```python
from build123d import *

# Parameters (mm, degrees)
F0_W     = 40
F0_H     = 20
F1_DEPTH = 6
F2_W     = 16
F2_H     = 12
F2_R     = 4.65
F3_DEPTH = 3
F4_DEPTH = 1.5
F5_SIZE  = 1


with BuildPart() as f1:
    # F0 (on Top) → F1 (new body)
    with BuildSketch(Plane.XY):
        with Locations((20, 10)):
            Rectangle(F0_W, F0_H)
    extrude(amount=F1_DEPTH)

    # F2 (on face) → F3 (cut)
    with BuildSketch(Plane.XY.offset(6)):
        with Locations((10, 10)):
            Rectangle(F2_W, F2_H)
        with Locations((12, 10)):
            Circle(F2_R, mode=Mode.SUBTRACT)
        with Locations((30, 10)):
            Rectangle(F2_W, F2_H)
        with Locations((32, 10)):
            Circle(F2_R, mode=Mode.SUBTRACT)
    extrude(amount=-F3_DEPTH, mode=Mode.SUBTRACT)

    # F4 (cut): faces of the model
    f4_faces = [f1.faces().sort_by_distance(p)[0] for p in [
        (12, 10, 6),
        (32, 10, 6),
    ]]
    extrude(f4_faces, amount=-F4_DEPTH, mode=Mode.SUBTRACT)

    # F5
    f5_edges = [f1.edges().sort_by_distance(p)[0] for p in [
        (10, 16, 6),
        (18, 10, 6),
        (10, 4, 6),
        (2, 10, 6),
        (22, 10, 6),
        (30, 16, 6),
        (38, 10, 6),
        (30, 4, 6),
    ]]
    chamfer(f5_edges, length=F5_SIZE)


solid = f1.part
```
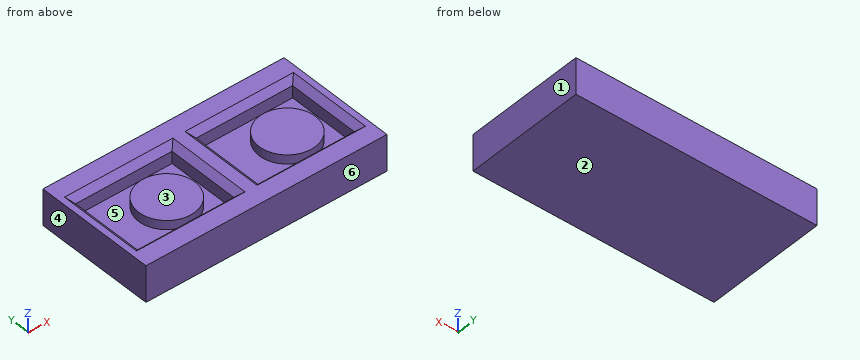
Could you check a few things on this model? Use its own coordinates, in mm. Face numbers are marked on the shaded views. A direction names the side the tool comes from. Coordinates: 2 decimals unless noted, no trailing zeros. Write each loop counter-clockwise with the first axis right and the second up, starting at its lowest first coordinate (ties: lowest second). Pieces come first, ordered by that corner, then holes. Notation, with made-up numbers: (1.25, 78) - (10.25, 78) arc R20 ccw to (10.25, 94) - close; hole circle Ø2 at (31, -30.75). An arc over 180 degrees is marked (long way). Use a Markdown table: item, result.
Q1. Thinking about a two-plate mould opening in X: for the marked faces 1, 2, 3 and 4, which applies, +X half, -X half, draft (parallel to the pull), parting line (faces both ways), or undercut?
Geometry check:
| item | result |
|---|---|
| face 1 | +X half |
| face 2 | draft |
| face 3 | undercut |
| face 4 | -X half |
Q2. Imagine slicing it at D-D (y = 10). List the corners of the cut face in (x, z) for me, and give its area (3 significant figures).
Geometry check:
| item | result |
|---|---|
| outline | (0, 0) - (40, 0) - (40, 6) - (39, 6) - (38, 5) - (38, 3) - (36.65, 3) - (36.65, 4.5) - (27.35, 4.5) - (27.35, 3) - (22, 3) - (22, 5) - (21, 6) - (19, 6) - (18, 5) - (18, 3) - (16.65, 3) - (16.65, 4.5) - (7.35, 4.5) - (7.35, 3) - (2, 3) - (2, 5) - (1, 6) - (0, 6) - close |
| area | 170 mm2 |
Q3. Please list where these lines run through material, in increasing order: L1, parallel to Y at x = 14, z = 3.25; L2, parallel to X at y = 12, z = 3.5; L3, parallel to Y at x = 4.5, z = 4.
Geometry check:
| item | result |
|---|---|
| L1 | y = 0 to 4, 5.8 to 14.2, 16 to 20 |
| L2 | x = 0 to 2, 7.8 to 16.2, 18 to 22, 27.8 to 36.2, 38 to 40 |
| L3 | y = 0 to 4, 16 to 20 |
Q4. I'm going to push a flat-ended pin straight in: pin 1 Ø6 at (x, y) = (28.5, 8.5) entering from +Z. Where does the tip first touch, or does it pass through?
Geometry check:
| item | result |
|---|---|
| pin 1 | stops at z = 4.5 |
Q5. Imagine slicing it at C-C (y = 3.5). List the corners of the cut face in (x, z) for me, and give its area (4 significant figures).
Geometry check:
| item | result |
|---|---|
| outline | (0, 0) - (40, 0) - (40, 6) - (39, 6) - (38.5, 5.5) - (21.5, 5.5) - (21, 6) - (19, 6) - (18.5, 5.5) - (1.5, 5.5) - (1, 6) - (0, 6) - close |
| area | 222.5 mm2 |
Q6. Which directions (+Z, -Z, +X, -X, +Y, -Y) give clear straight access to the entire face, cutting with the end or side of a thin tool? Please do the marked faces 5 and 6.
Geometry check:
| item | result |
|---|---|
| face 5 | +Z |
| face 6 | +Z, -Z, +X, -X, -Y |
Q7. Imagine slicing it at B-B (x = 24.5). List the corners of the cut face in (y, z) for me, and give its area (3 significant figures).
Geometry check:
| item | result |
|---|---|
| outline | (0, 0) - (20, 0) - (20, 6) - (17, 6) - (16, 5) - (16, 3) - (4, 3) - (4, 5) - (3, 6) - (0, 6) - close |
| area | 83.0 mm2 |
Q8. Imagine slicing it at A-A (z = 3.5). List the corners of the cut face in (x, y) for me, and give its area (3 significant figures).
Geometry check:
| item | result |
|---|---|
| outline | (0, 0) - (40, 0) - (40, 20) - (0, 20) - close; circle Ø9.3 at (12, 10); circle Ø9.3 at (32, 10); hole (2, 4) - (18, 4) - (18, 16) - (2, 16) - close; hole (22, 4) - (38, 4) - (38, 16) - (22, 16) - close |
| area | 552 mm2 |
